Design review of the part shown in the three views and the two pictorial views. Dimensions are in mm from the part's minimum x, y and z. Coordinates: 2 decimals unless noted, no trailing zeros. Loops run counter-clockwise (first coordinate to the right, second up) from the corner with the lowest first, then second, coordinate; pieces in that order, holes last. Notation, with made-up numbers: M 71,11 L 92,11 A23 ccw 92,28 Z; hole C 74,3.5 d3. An arc over 180 degrees is marked long. Use one line per item in the form item = value.
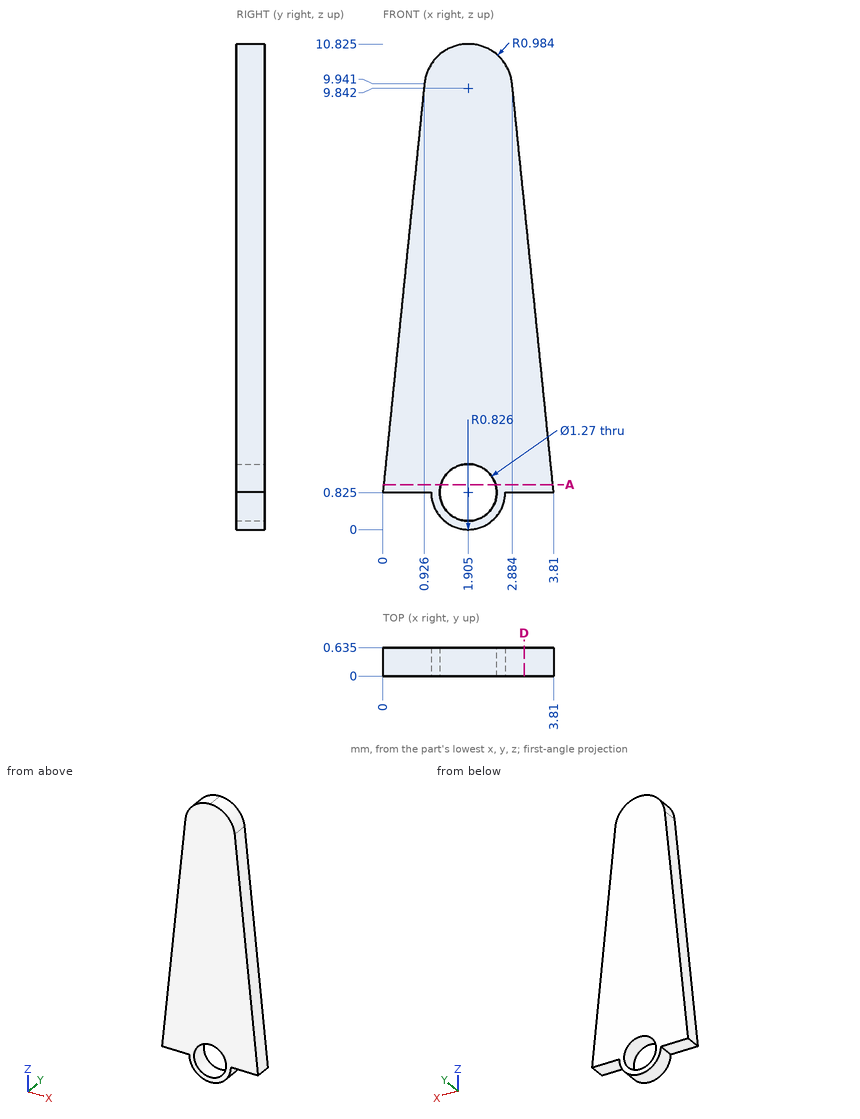
1. Add section D-D (x = 3.15). State the section outline as (y, z) points (1 decimal).
Response values:
outline = M 0,0.8 L 0.6,0.8 L 0.6,7.3 L 0,7.3 Z
2. Wall thickness on line 1 along Z through (x, y) = (2.35, 0.05) (1 decimal); line 2 along Z through (x, y) = (2.2, 0.55) (1 decimal); line 3 along X through (y, z) = (0.1, 1.25) (1 decimal): over which ranges is each line inside the solid? List them lowest first. Write a range as from..to.
Response values:
line_1 = 0.1..0.4, 1.3..10.7
line_2 = 0.1..0.3, 1.4..10.8
line_3 = 0..1.4, 2.4..3.8
3. Insertion check: P1, Ø1, axis at x = 1.9, z = 0.83, coming from the +Y side. The pin has a flat end and moves straight along its axis. Give the tip position at first contact, or say it passes through.
Response values:
P1 = through
4. Add section A-A (z = 1). State the section outline as (x, y) points (1 decimal).
Response values:
outline = M 0,0 L 1.3,0 L 1.3,0.6 L 0,0.6 Z; M 2.5,0 L 3.8,0 L 3.8,0.6 L 2.5,0.6 Z
